from build123d import *

# Parameters (mm, degrees)
CROQUIS1_R              = 16
CROQUIS1_R_2            = 12.5
SALIENTE_EXTRUIR1_DEPTH = 2
CHAFL_N1_SIZE           = 0.5
CROQUIS2_R              = 14.793460403
CROQUIS2_R_2            = 13.590473759
SALIENTE_EXTRUIR2_DEPTH = 2.05


with BuildPart() as part:
    # Croquis1 → Saliente-Extruir1 (new body, symmetric)
    with BuildSketch(Plane(origin=(0, 0, 0), x_dir=(1, 0, 0), z_dir=(0, 1, 0))):
        Circle(CROQUIS1_R)
        Circle(CROQUIS1_R_2, mode=Mode.SUBTRACT)
    extrude(amount=SALIENTE_EXTRUIR1_DEPTH, both=True)

    # Chaflán1
    chafl_n1_edges = [part.edges().sort_by_distance(p)[0] for p in [
        (-16, -2, 0),
        (-16, 2, 0),
        (-12.5, -2, 0),
        (-12.5, 2, 0),
    ]]
    chamfer(chafl_n1_edges, length=CHAFL_N1_SIZE)

    # Croquis2 → Saliente-Extruir2 (add, symmetric)
    with BuildSketch(Plane(origin=(0, 0, 0), x_dir=(1, 0, 0), z_dir=(0, 1, 0))):
        Circle(CROQUIS2_R)
        Circle(CROQUIS2_R_2, mode=Mode.SUBTRACT)
    extrude(amount=SALIENTE_EXTRUIR2_DEPTH, both=True)


solid = part.part
Verification items for the finished model (mm, model axes). A direction names the side the tool comes from. Round coordinates to 2 decimals unless told otherwise and drop trailing zeros. Order: outer loops, then holes, each group sorted by start corner. A loop starts at its lowest first (then second) coordinate and runs counter-clockwise, first axis right, second up.
1. Release check for a two-part mould opening along Z. For faces 1 (the cylindrical face through (-3.47, 0.02, 15.62)), 2 (the flat face through (7, -2.05, 12)), 3 (the cylindrical face through (11.923, -0.021, -3.755)) record: +Z half, -Z half, draft (parallel to the pull), parting line (faces both ways), or undercut.
Final values:
face 1: parting line
face 2: draft
face 3: undercut
2. Access from +Z, -Z, +X, -X, +Y, -Y to the whole of each face (thin tool, end or side, straight path). Record for faces 4 (the flat face through (14, 2, 6)), 5 (the flat face through (14, -2, 6)), 6 (the flat face through (7, 2.05, 12)).
Final values:
face 4: +Y
face 5: -Y
face 6: +Z, -Z, +X, -X, +Y
3. Thickness scan on L1, parallel to Z at x = 0, y = 1.2; L2, parallel to X at y = 1.4, z = 10.5. Record the ranges inside material, lowest first.
Final values:
L1: z = -16 to -12.5, 12.5 to 16
L2: x = -12.07 to -6.78, 6.78 to 12.07
4. Go/stop test with flat-tipped pins: P1, Ø6, axis at x = -7, z = 4, coming from the -Y side; P2, Ø2, axis at y = -1, z = -2, coming from the +X side; P3, Ø3, axis at x = -10.5, z = -12.5, coming from the -Y side. Record where each tip stops, or that it passes through.
Final values:
P1: passes through
P2: stops at x = 15.97
P3: stops at y = -2
5. Section check C-C on y = -0.35. Record the cut outline in (x, z).
Final values:
outline: circle Ø32 at (0, 0); hole circle Ø25 at (0, 0)
